Verification items for the finished model (mm, model axes). Give positions to 0.01 mm unless a question says otherwise; leave off trailing zeros. Order: outer loops, then holes, each group sorted by start corner. A loop starts at its lowest first (then second) coordinate and runs counter-clockwise, first axis right, second up. Notation, with made-up numbers: (29.5, -6.5) - (88.5, -6.5) arc R23 cw to (88.5, 15.5) - close; hole circle Ø8 at (-26, -34). An arc over 180 degrees is marked (long way). Answer as a JSON object with one key per item and string values. Group by question number.
(1) Section check C-C (y = 3.25). Record the boundary of the cut face in (x, z).
(2) Section check A-A (x = 5). Record the boundary of the cut face in (y, z), then the cut area to 3 significant figures.
(3) Thickness scan on line 1 (Y direction, x = 45.5, z = 134); line 2 (Y direction, x = 37.5, z = 72). Record the ranges inside material, lowest first.
(4) Depth check by flat-ended pin: pin 1 Ø10 at (x, y) = (42.5, 16.5) entering from -Z; pin 2 Ø4 at (x, y) = (18.5, 16.5) entering from -Z; pin 3 Ø1 at (x, z) = (24.5, 82.5) entering from +Y. Enter the tip coordinate at first touch or a pass-through.
(5) Section check B-B (z = 79.5). Record the boundary of the cut face in (x, y), then the cut area to 3 significant figures.
Autodesk Inventor part; units mm, degrees
ref_plane "YZ Plane" through (0, 0, 0) normal (1, 0, 0) x (0, 1, 0)
ref_plane "XZ Plane" through (0, 0, 0) normal (0, 1, 0) x (-1, 0, 0)
ref_plane "XY Plane" through (0, 0, 0) normal (0, 0, 1) x (1, 0, 0)
sketch "Sketch1" plane through (0, 0, 0) normal (0, 0, 1) x (1, 0, 0)
  line L0 (0, 0) -> (50.8, 0)
  line L1 (50.8, 0) -> (50.8, 50.8)
  line L2 (50.8, 50.8) -> (0, 50.8)
  line L3 (0, 50.8) -> (0, 0)
  dimension "d0" = 50.8
  dimension "d1" = 50.8
extrude "Extrusion1" add sketch "Sketch1" along normal blind 127
sketch "Sketch2" plane through (50.8, 0, 0) normal (1, 0, 0) x (0, 0, -1)
  line L0 (-127, 50.8) -> (-127, 0)
  line L1 (0, 0) -> (-127, 0)
  line L2 (0, 0) -> (0, 50.8)
  line L3 (0, 50.8) -> (-127, 50.8)
  line L4 (-127, 0) -> (-66.6079, 19.6226)
  line L5 (-127, 0) -> (-63.5, 0) construction
  line L6 (-66.6079, 19.6226) -> (-60.2321, 0)
  line L7 (-60.2321, 0) -> (-127, 0)
  dimension "d4" = 63.5
  dimension "d5" = 18
extrude "Extrusion2" cut sketch "Sketch2" against normal blind 127 contours L3 L2 L1 L6 L4 L0
sketch "Sketch3" plane through (50.8, 0, 127) normal (1, 0, 0) x (0, 0, -1)
  line L0 (66.7679, 0) -> (60.3921, 19.6226)
  line L1 (60.3921, 19.6226) -> (0, 0)
  line L2 (66.7679, 0) -> (0, 0)
  line L3 (60.3921, 19.6226) -> (-12.0784, -3.9245)
  line L4 (-12.0784, -3.9245) -> (70.1883, -3.9245)
  line L5 (60.3921, 19.6226) -> (68.043, -3.9245)
  point P0 (127, 0)
  dimension "d8" = 76.2
extrude "Extrusion3" add sketch "Sketch3" against normal blind 50.8 contours L5 L4 L3 L2
properties part number "Goal Guide 2"
Solutions:
{
 "1": {"outline": "(0, 61.29) - (50.8, 61.29) - (50.8, 117) - (0, 117) - close"},
 "2": {"outline": "(-3.92, 58.96) - (0, 60.23) - (19.62, 66.61) - (0, 127) - (-3.92, 139.08) - close", "area": "943 mm2"},
 "3": {"line 1": "y = -3.92 to -2.27", "line 2": "y = -3.92 to 17.87"},
 "4": {"pin 1": "stops at z = 63.97", "pin 2": "stops at z = 64.94", "pin 3": "stops at y = 14.62"},
 "5": {"outline": "(0, -3.92) - (50.8, -3.92) - (50.8, 15.43) - (0, 15.43) - close", "area": "983 mm2"}
}
